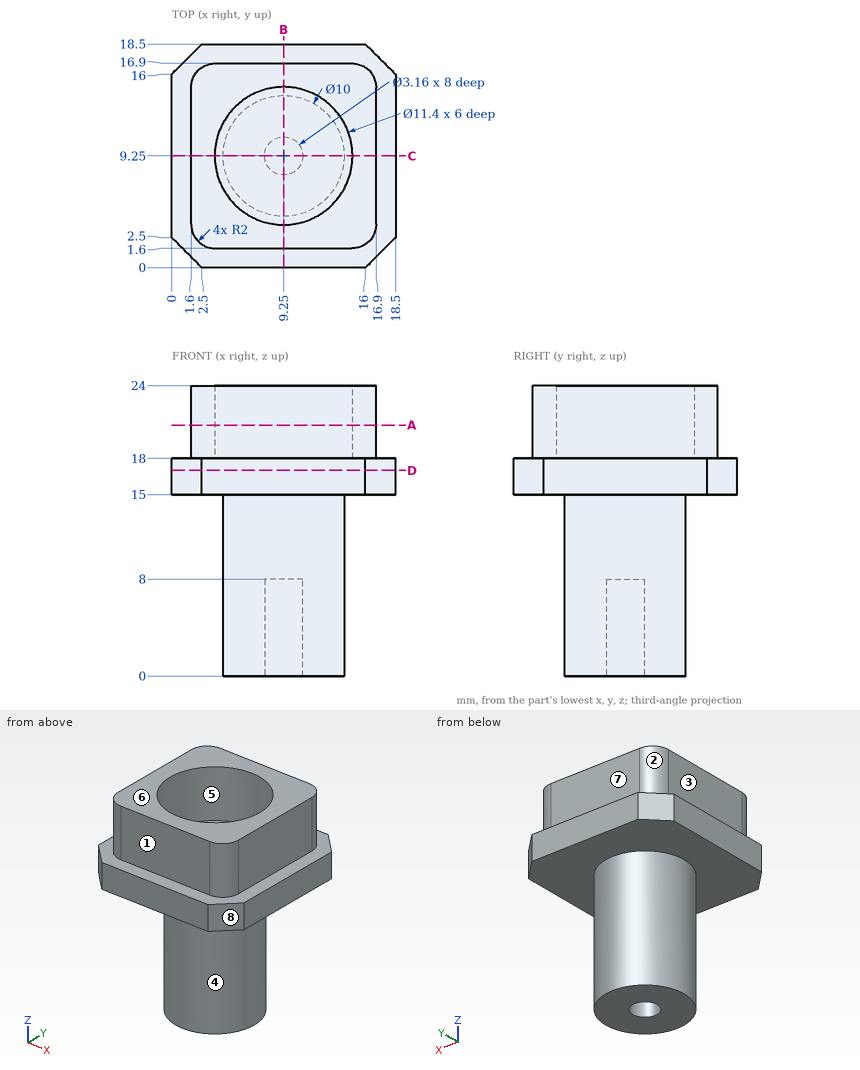
Can you work these out from the drawing? Everything is in mm from the part's minimum corner. A direction names the side the tool comes from. Round coordinates to 2 decimals unless told otherwise and drop trailing zeros. Write each loop counter-clockwise with the first axis right and the second up, starting at its lowest first coordinate (ties: lowest second). Pieces come first, ordered by that corner, then holes. Notation, with made-up numbers: (29.5, -20.75) - (45.5, -20.75) arc R23 cw to (45.5, 8.25) - close; hole circle Ø1 at (35, 79.5). An arc over 180 degrees is marked (long way). Write each question's results on one line, items separated by ' | '. Start each with the question number.
1) Which directions (+Z, -Z, +X, -X, +Y, -Y) give clear straight access to the entire face, cutting with the end or side of a thin tool? Please do the marked faces 1, 2, 3 and 4.
2) Suppose I cut it at B-B (x = 9.25). List the corners of the cut face in (y, z) for me.
3) For pin 1 Ø3 at (x, y) = (6, 2) entering from -Z; pin 2 Ø1.8 at (x, z) = (9, 20) entering from -Y; pin 3 Ø5 at (x, z) = (8.5, 22.5) entering from +Y, each with a flat end and sliding along its axis, tell me the tip position at first contact or that it passes through.
4) We'd pull the mould along Y, two halves only. Please class the marked faces 5, 6, 7 and 8: released by +Y, released by -Y, zero draft, split by the parting line, or undercut.
5) Please list where these lines run through material, in increasing order: line 1 (Y direction, x = 9.25, z = 5.25); line 2 (Z direction, x = 9.75, y = 17.5).
6) Suppose I cut it at A-A (z = 20.75). List the corners of the cut face in (x, y) for me.
7) Suppose I cut it at D-D (z = 17). List the corners of the cut face in (x, y) for me, and give its area (3 significant figures).
Here are the results:
1) face 1: +Z, +X, -X, -Y | face 2: +Z, -X, +Y | face 3: +Z, -X, +Y, -Y | face 4: -Z
2) outline: (0, 15) - (4.25, 15) - (4.25, 0) - (7.67, 0) - (7.67, 8) - (10.83, 8) - (10.83, 0) - (14.25, 0) - (14.25, 15) - (18.5, 15) - (18.5, 18) - (16.9, 18) - (16.9, 24) - (14.95, 24) - (14.95, 18) - (3.55, 18) - (3.55, 24) - (1.6, 24) - (1.6, 18) - (0, 18) - close
3) pin 1: stops at z = 15 | pin 2: stops at y = 1.6 | pin 3: stops at y = 16.9
4) face 5: undercut | face 6: zero draft | face 7: released by +Y | face 8: released by -Y
5) line 1: y = 4.25 to 7.67, 10.83 to 14.25 | line 2: z = 15 to 18
6) outline: (1.6, 3.6) arc R2 ccw to (3.6, 1.6) - (14.9, 1.6) arc R2 ccw to (16.9, 3.6) - (16.9, 14.9) arc R2 ccw to (14.9, 16.9) - (3.6, 16.9) arc R2 ccw to (1.6, 14.9) - close; hole circle Ø11.4 at (9.25, 9.25)
7) outline: (0, 2.5) - (2.5, 0) - (16, 0) - (18.5, 2.5) - (18.5, 16) - (16, 18.5) - (2.5, 18.5) - (0, 16) - close | area: 330 mm2
